Input: part model. Units: mm. Frame: model coordinates. Face numbers are marked on the shaded views. Give positions to 0.01 mm unless a question says otherwise; leave off trailing zeros. Loops run counter-clockwise (first coordinate to the right, second up) from the corner with the lowest first, then second, coordinate; pieces in that order, holes last. Notation, with made-up numbers: M 53,48 L 79,48 A14 ccw 79,60 Z; hole C 16.5,80 d1. An arc over 180 degrees is marked long. Use CSV: the item, a comma, the result in double quotes. Start each with the question number.
Q1. Section C-C, the plane z = 11. Output: boundary loops of the cut face in (x, y), plus the area to 3 significant figures.
Q2. Section A-A, the plane y = 0. Output: boundary loops of the cut face in (x, z).
Q3. Pin query (flat end, axial travel): pin 1 (6 mm diameter, centred on x = 5, z = 8.5, fed in from +Y); pin 2 (1 mm diameter, centred on x = -1, z = 14, fed in from +Y); pin 3 (1.5 mm diameter, centred on x = 1.5, y = -7, fed in from +Z). Return the tip coordinate at first contact, or that it passes through.
Q4. Pull-direction query (Y, two-part tool) for the marked faces 1, 2 and 3; classes: released by +Y, released by -Y, zero draft, split by the parting line, or undercut.
Q5. Material intervals for line 1 along Y through (x, z) = (0, 5.75); line 2 along X through (y, z) = (-0.25, 4.75); line 3 along X through (y, z) = (0.25, 9.25), sorted ascending.
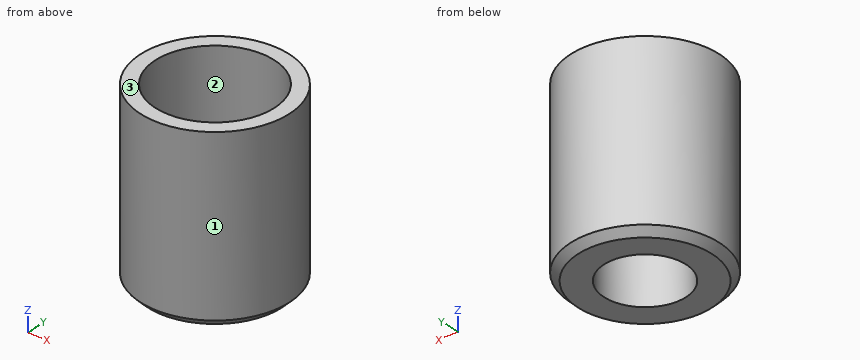
from build123d import *

# Parameters (mm, degrees)
F0_R     = 10
F1_DEPTH = 24
F2_SIZE  = 1
F3_R     = 5.5
F4_DEPTH = 24.001
F5_R     = 8
F6_DEPTH = 16


with BuildPart() as f1:
    # F0 (on Top) → F1 (new body)
    with BuildSketch(Plane.XY):
        Circle(F0_R)
    extrude(amount=F1_DEPTH)

    # F2
    f2_edges = [f1.edges().sort_by_distance(p)[0] for p in [
        (-10, 0, 0),
    ]]
    chamfer(f2_edges, length=F2_SIZE)

    # F3 (on face) → F4 (cut, through all)
    with BuildSketch(Plane.XY.offset(24)):
        Circle(F3_R)
    extrude(amount=-F4_DEPTH, mode=Mode.SUBTRACT)

    # F5 (on face) → F6 (cut)
    with BuildSketch(Plane.XY.offset(24)):
        Circle(F5_R)
    extrude(amount=-F6_DEPTH, mode=Mode.SUBTRACT)


solid = f1.part
A:
1,outline,"C 0,0 d20; hole C 0,0 d16"
1,area,"113 mm^2"
2,outline,"M -10,1 L -9,0 L -5.5,0 L -5.5,8 L -8,8 L -8,24 L -10,24 Z; M 5.5,0 L 9,0 L 10,1 L 10,24 L 8,24 L 8,8 L 5.5,8 Z"
3,pin 1,"y = 9.8"
3,pin 2,"y = 9.99"
3,pin 3,"z = 8"
4,face 1,"split by the parting line"
4,face 2,"undercut"
4,face 3,"zero draft"
5,line 1,"-10 to -5.5, 5.5 to 10"
5,line 2,"-10 to -5.49, 5.49 to 10"
5,line 3,"-10 to -8, 8 to 10"
